For this review, take the finished solid that the model builds, in its own axes (mm). Face numbers are marked on the shaded views. Coordinates: 2 decimals unless noted, no trailing zeros. Loops run counter-clockwise (first coordinate to the right, second up) from the corner with the lowest first, then second, coordinate; pieces in that order, holes last. Notation, with made-up numbers: M -20.5,-29.75 L 38.5,-29.75 A7 ccw 38.5,-19.75 Z; hole C -18.5,88 d2. An arc over 180 degrees is marked long. Answer as a JSON object with one key per item and string values. Group by question number.
Item 1: Wall thickness on L1, parallel to Y at x = 0, z = 1; L2, parallel to Y at x = 5.5, z = 0.95; L3, parallel to Y at x = 4, z = 1.05: over which ranges is each line inside the solid? List them lowest first. Write a range as from..to.
Item 2: Mouldability with a two-part tool opening along Y and no side actions: class the marked faces 1, 2 and 3 as +Y half, -Y half, draft (parallel to the pull), parting line (faces both ways), or undercut.
Item 3: Insertion check: pin 1 (1.9 mm diameter, centred on x = 0, y = -5.5, fed in from +Z); pin 2 (1.9 mm diameter, centred on x = 0, y = 0, fed in from +Z). Each pin has a flat end and moves straight along its axis. Give the tip position at first contact, or say it passes through.
Item 4: Add section B-B (x = 0). State the section outline as (y, z) points.
Item 5: Add section A-A (y = 0). State the section outline as (x, z) points.
Item 6: Add section C-C (z = 0.7). State the section outline as (x, y) points, then the cut area to 3 significant figures.
Item 7: Add section D-D (y = 3). State the section outline as (x, z) points.
from build123d import *

# Parameters (mm, degrees)
F0_R     = 8.3
F1_DEPTH = 1.25
F2_R     = 1.05
F3_DEPTH = 25
F4_R     = 1.05
F5_DEPTH = 0.75


with BuildPart() as f1:
    # F0 (on Top) → F1 (new body)
    with BuildSketch(Plane.XY):
        Circle(F0_R)
    extrude(amount=F1_DEPTH)

    # F2 (on face) → F3 (cut)
    with BuildSketch(Plane.XY.offset(1.25)):
        Circle(F2_R)
    extrude(amount=-F3_DEPTH, mode=Mode.SUBTRACT)

    # F4 (on face) → F5 (cut)
    with BuildSketch(Plane.XY.offset(1.25)):
        with Locations((0, 5.5)):
            Circle(F4_R)
        with Locations((-4.76314, 2.75)):
            Circle(F4_R)
        with Locations((-4.76314, -2.75)):
            Circle(F4_R)
        with Locations((0, -5.5)):
            Circle(F4_R)
        with Locations((4.76314, -2.75)):
            Circle(F4_R)
        with Locations((4.76314, 2.75)):
            Circle(F4_R)
    extrude(amount=-F5_DEPTH, mode=Mode.SUBTRACT)


solid = f1.part
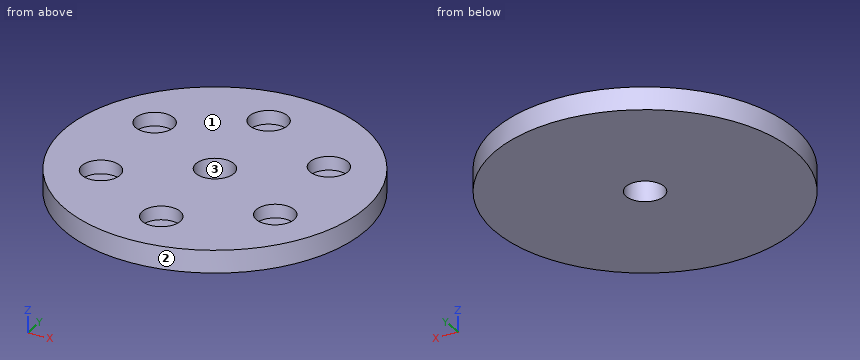
From the geometry:
{
 "1": {"L1": "y = -8.3..-6.55, -4.45..-1.05, 1.05..4.45, 6.55..8.3", "L2": "y = -6.22..-3.5, -2..2, 3.5..6.22", "L3": "y = -7.27..-3.47, -2.03..2.03, 3.47..7.27"},
 "2": {"face 1": "draft", "face 2": "parting line", "face 3": "undercut"},
 "3": {"pin 1": "stops at z = 0.5", "pin 2": "passes through"},
 "4": {"outline": "M -8.3,0 L -1.05,0 L -1.05,1.25 L -4.45,1.25 L -4.45,0.5 L -6.55,0.5 L -6.55,1.25 L -8.3,1.25 Z; M 1.05,0 L 8.3,0 L 8.3,1.25 L 6.55,1.25 L 6.55,0.5 L 4.45,0.5 L 4.45,1.25 L 1.05,1.25 Z"},
 "5": {"outline": "M -8.3,0 L -1.05,0 L -1.05,1.25 L -8.3,1.25 Z; M 1.05,0 L 8.3,0 L 8.3,1.25 L 1.05,1.25 Z"},
 "6": {"outline": "C 0,0 d16.6; hole C -4.76,-2.75 d2.1; hole C -4.76,2.75 d2.1; hole C 0,-5.5 d2.1; hole C 0,0 d2.1; hole C 0,5.5 d2.1; hole C 4.76,-2.75 d2.1; hole C 4.76,2.75 d2.1", "area": "192 mm²"},
 "7": {"outline": "M -7.74,0 L 7.74,0 L 7.74,1.25 L 5.78,1.25 L 5.78,0.5 L 3.74,0.5 L 3.74,1.25 L -3.74,1.25 L -3.74,0.5 L -5.78,0.5 L -5.78,1.25 L -7.74,1.25 Z"}
}
